Read the model definition and answer for the solid it produces. Units are mm, in the model's axes. A direction names the side the tool comes from. Round coordinates to 2 decimals unless told otherwise and drop trailing zeros. Write each loop counter-clockwise with the first axis right and the second up, starting at its lowest first coordinate (ties: lowest second). Pieces come first, ordered by that corner, then holes. Notation, with made-up numbers: (49, 79.25) -> (70, 79.25) arc R16 ccw to (70, 102.25) -> close; hole circle Ø11 at (-25, -21). An arc over 180 degrees is marked (long way). Return JSON: item names as keys, results as strings.
Autodesk Inventor part; units mm, degrees
ref_plane "YZ Plane" through (0, 0, 0) normal (1, 0, 0) x (0, 1, 0)
ref_plane "XZ Plane" through (0, 0, 0) normal (0, 1, 0) x (-1, 0, 0)
ref_plane "XY Plane" through (0, 0, 0) normal (0, 0, 1) x (1, 0, 0)
sketch "Sketch1" plane through (0, 0, 0) normal (0, 0, 1) x (1, 0, 0)
  line L0 (0, 0) -> (20, 0)
  line L1 (20, 0) -> (20, 60)
  line L2 (20, 60) -> (0, 60)
  line L3 (0, 60) -> (0, 0)
  dimension "d0" = 20
  dimension "d1" = 60
extrude "Extrusion1" add sketch "Sketch1" along normal blind 15
fillet "Fillet1" radius 7 2 edges at (20, 60, 7.5) (20, 0, 7.5)
sketch "Sketch2" plane through (0, 0, 15) normal (0, 0, 1) x (1, 0, 0)
  arc A0 (20, 53) -> (13, 60) centre (13, 53) ccw
  line L0 (13, 60) -> (13, 32.5)
  line L1 (13, 60) -> (13, 47)
  arc A1 (13, 0) -> (20, 7) centre (13, 7) ccw
  line L2 (13, 0) -> (13, 13)
  line L3 (13, 47) -> (4, 47) construction
  line L4 (13, 45) -> (4, 45)
  line L5 (4, 49) -> (13, 49)
  arc A2 (13, 45) -> (13, 49) centre (13, 47) ccw
  arc A3 (4, 49) -> (4, 45) centre (4, 47) ccw
  line L6 (13, 13) -> (4, 13) construction
  line L7 (13, 11) -> (4, 11)
  line L8 (4, 15) -> (13, 15)
  arc A4 (13, 11) -> (13, 15) centre (13, 13) ccw
  arc A5 (4, 15) -> (4, 11) centre (4, 13) ccw
  line L9 (13, 60) -> (0, 60)
  line L10 (13, 60) -> (13, 30)
  circle A6 centre (13, 30) radius 2.5
  point P0 (0, 0)
  point P1 (8.5, 47)
  point P2 (8.5, 13)
  dimension "d5" = 27.5
  dimension "d7" = 13
  dimension "d8" = 13
  dimension "d13" = 30
  dimension "d14" = 5
extrude "Extrusion2" cut sketch "Sketch2" against normal through all
sketch "Sketch3" plane through (20, 7, 0) normal (1, 0, 0) x (0, 0, -1)
  line L0 (-14, 0) -> (-14, 46)
  line L1 (-14, 0) -> (-6, 0)
  line L2 (-6, 0) -> (-6, 46)
  line L3 (-6, 46) -> (-14, 46)
  line L4 (-14, 46) -> (-14, 0)
  point P0 (0, -7)
extrude "Extrusion3" cut sketch "Sketch3" against normal blind 20
sketch "Sketch4" plane through (0, 0, 15) normal (0, 0, 1) x (1, 0, 0)
  point P0 (0, 0)
sketch "Sketch5" plane through (0, 0, 15) normal (0, 0, 1) x (1, 0, 0)
  point P0 (0, 0)
sketch "Sketch6" plane through (20, 7, 14) normal (0, 0, -1) x (-1, 0, 0)
  line L0 (0, 46) -> (0, 0)
  line L1 (0, 0) -> (20, 0)
  line L2 (20, 0) -> (20, 46)
  line L3 (20, 46) -> (0, 46)
  line L4 (0, 46) -> (0, 0)
  point P0 (20, -7)
extrude "Extrusion4" add sketch "Sketch6" along normal blind 3
sketch "Sketch7" plane through (0, 0, 15) normal (0, 0, 1) x (1, 0, 0)
  circle A0 centre (13, 30) radius 2.5
  point P0 (0, 0)
extrude "Extrusion5" cut sketch "Sketch7" against normal through all
sketch "Sketch8" plane through (0, 0, 15) normal (0, 0, 1) x (1, 0, 0)
  arc A0 (13, 11) -> (13, 15) centre (13, 13) ccw
  line L0 (13, 11) -> (4, 11)
  line L1 (13, 11) -> (4, 11)
  line L2 (4, 11) -> (4, 11)
  line L3 (4, 11) -> (13, 11)
  line L4 (13, 11) -> (13, 11)
  arc A1 (13, 45) -> (13, 49) centre (13, 47) ccw
  line L5 (4, 45) -> (13, 45)
  line L6 (13, 45) -> (13, 45)
  line L7 (13, 45) -> (4, 45)
  line L8 (4, 45) -> (4, 45)
  line L9 (4, 45) -> (13, 45)
  arc A2 (13, 45) -> (13, 49) centre (13, 47) ccw
  arc A3 (4, 49) -> (4, 45) centre (4, 47) ccw
  arc A4 (4, 49) -> (4, 45) centre (4, 47) ccw
  arc A5 (13, 11) -> (13, 15) centre (13, 13) ccw
  arc A6 (4, 15) -> (4, 11) centre (4, 13) ccw
  line L10 (4, 15) -> (13, 15)
  line L11 (4, 15) -> (13, 15)
  line L12 (4, 49) -> (13, 49)
  line L13 (4, 49) -> (13, 49)
  arc A7 (4, 49) -> (4, 45) centre (4, 47) ccw
  line L14 (13, 45) -> (4, 45)
  arc A8 (4, 15) -> (4, 11) centre (4, 13) ccw
  arc A9 (4, 15) -> (4, 15) centre (4, 13) ccw
  point P0 (0, 0)
extrude "Extrusion6" cut sketch "Sketch8" against normal through all
sketch "Sketch9" plane through (20, 7, 6) normal (0, 0, 1) x (1, 0, 0)
  line L0 (0, 46) -> (-20, 46)
  arc A0 (-7, -7) -> (0, 0) centre (-7, 0) ccw
  line L1 (-20, 46) -> (0, 46)
  line L2 (0, 46) -> (0, 0)
  line L3 (0, 0) -> (-20, 0)
  line L4 (-20, 0) -> (-20, 46)
  point P0 (-20, -7)
extrude "Extrusion7" cut sketch "Sketch9" against normal blind 2
properties part number "3C_LiPoBatteryHolder_mountingBracket"
Item 1: Section A-A (y = 30) is taken. Give the vertices of the cut face in (x, z), then the cut area to 3 significant figures.
Worked answers:
{"outline": "(0, 0) -> (10.5, 0) -> (10.5, 4) -> (0, 4) -> close; (0, 11) -> (10.5, 11) -> (10.5, 15) -> (0, 15) -> close; (15.5, 0) -> (20, 0) -> (20, 4) -> (15.5, 4) -> close; (15.5, 11) -> (20, 11) -> (20, 15) -> (15.5, 15) -> close", "area": "120 mm2"}
Item 2: Section C-C (x = 14.25) is taken. State how many separate pieces and enclosed holes the cut face has, then the cut area to 3 significant figures.
Worked answers:
{"separate pieces": "6", "enclosed holes": "0", "area": "490 mm2"}
Item 3: A tool of negligible diameter and unlimited length cuts with its end or side. For faces 1 (the flat face through (8, 49, 2)), 2 (the flat face through (10, 30, 11)), 3 (the cylindrical face through (18, 57.9, 7.6)), from which of +Z, -Z, +X, -X, +Y, -Y can it reach the whole face along a straight path? Write none if from no direction.
Worked answers:
{"face 1": "+Z, -Z", "face 2": "+X, -X", "face 3": "+Z, -Z, +X, +Y"}
Item 4: Straight lines are drawn through the part: L1, parallel to Y at x = 6.25, z = 1.25; L2, parallel to Y at x = 13, z = 12.25; L3, parallel to Z at x = 2.25, y = 36. For each, find the intervals that lie inside material, in ascending order. Write a range as [from, to].
Worked answers:
{"L1": "y = [0, 11], [15, 45], [49, 60]", "L2": "y = [0, 11], [15, 27.5], [32.5, 45], [49, 60]", "L3": "z = [0, 4], [11, 15]"}
Item 5: Section D-D (y = 13) is taken. Give the vertices of the cut face in (x, z).
Worked answers:
{"outline": "(0, 0) -> (2, 0) -> (2, 4) -> (0, 4) -> close; (0, 11) -> (2, 11) -> (2, 15) -> (0, 15) -> close; (15, 0) -> (20, 0) -> (20, 4) -> (15, 4) -> close; (15, 11) -> (20, 11) -> (20, 15) -> (15, 15) -> close"}
Item 6: Section B-B (z = 13.75) is taken. Give the vertices of the cut face in (x, y), then the cut area to 3 significant figures.
Worked answers:
{"outline": "(0, 0) -> (13, 0) arc R7 ccw to (20, 7) -> (20, 53) arc R7 ccw to (13, 60) -> (0, 60) -> close; hole (4, 11) -> (13, 11) arc R2 ccw to (13, 15) -> (4, 15) arc R2 ccw to start; hole (4, 45) -> (13, 45) arc R2 ccw to (13, 49) -> (4, 49) arc R2 ccw to start; hole circle Ø5 at (13, 30)", "area": "1,060 mm2"}
Item 7: Flat-ended cylindrical pins translate along their axes: pin 1 (5 mm diameter, centred on x = 16.5, z = 1.5, fed in from -Y); pin 2 (1 mm diameter, centred on x = 15.5, z = 2, fed in from -Y); pin 3 (8 mm diameter, centred on x = 17.5, z = 12.5, fed in from +Y). Find the tip coordinate at first contact, or state that the pin passes through.
Worked answers:
{"pin 1": "stops at y = 0.07", "pin 2": "stops at y = 0.29", "pin 3": "stops at y = 59.98"}
Item 8: For a pull along X with two mould halves and no side action, classify faces 4 (the flat face through (20, 30, 2)), 5 (the flat face through (8, 15, 13)), 6 (the flat face through (10, 30, 0)) as released by +X, released by -X, zero draft, split by the parting line, or undercut.
Worked answers:
{"face 4": "released by +X", "face 5": "undercut", "face 6": "zero draft"}
